Read the model definition and answer for the solid it produces. Units are mm, in the model's axes. A direction names the side the tool comes from. Coordinates: 2 decimals unless noted, no trailing zeros. Loops run counter-clockwise (first coordinate to the right, second up) from the corner with the lowest first, then second, coordinate; pieces in that order, holes last. Notation, with made-up numbers: (30, -10) -> (42, -10) arc R26 ccw to (42, 14) -> close; hole circle Ø11 at (-6.5, -18.75). An arc over 180 degrees is marked (long way). Answer as a JSON object with one key per item and string values. Group by question number.
1) Consider probe 1 along Z at (x, y) = (66.25, -11); probe 2 along Z at (x, y) = (66.5, -12.5); probe 3 along Y at (x, z) = (70.75, 12.5). Determine where each line is inside the solid, lowest interval first. Write a range as [from, to].
2) Section A-A, the plane z = -61.5 is taken. Give the vertices of the cut face in (x, y), plus the area to 3 significant figures.
3) Section C-C, the plane z = -37.5 is taken. Give the vertices of the cut face in (x, y), plus the area to 3 significant figures.
4) Which of the six approach directions +Z, -Z, +X, -X, +Y, -Y give full straight-line access (tool end or side, diameter ignored) to faces 1 (the face through (67.438, -19.529, -39.122)), 2 (the face through (71, -18, -17.546)), 3 (the face through (69.563, -27.304, -67.9))?
5) Flat-ended cylindrical pins translate along their axes: P1, Ø2, axis at x = 69.5, y = -17.5, coming from the +Z side; P2, Ø1.5, axis at x = 67, z = -55, coming from the -Y side; P3, Ø1.5, axis at x = 69, z = -9.5, coming from the -Y side. Find the tip coordinate at first contact, or state that the pin passes through.
6) Determine the mould class of faces 4 (the face through (69, 0, 5)), 5 (the face through (71, -19.393, -2)) for opening direction Z: released by +Z, released by -Z, zero draft, split by the parting line, or undercut.
7) Section B-B, the plane y = -21 is taken. Give the vertices of the cut face in (x, z), plus the area to 3 significant figures.
from build123d import *

# Parameters (mm, degrees)
F1_DEPTH    = 37
F2_T1_DEPTH = 342.8505669038
F3_T        = -2.54
F4_W        = 125.55387271
F4_H        = 111.9176980871
F5_DEPTH    = 25.4
F6_R        = 3.175
F7_DEPTH    = 19.05
F9_DEPTH    = 142.24
F10_W       = 3.5
F10_H       = 32
F11_DEPTH   = 5
F12_W       = 142.5411626697
F12_H       = 154.7065079212
F13_DEPTH   = 37.001


# Not quite as in the source:
# - a fillet or chamfer that OpenCascade refuses, or shapes differently, is made with other operations: its cross-section is extruded or revolved along the edge and cut away or added


with BuildPart() as f1:
    # F0 (on Front) → F1 (new body)
    with BuildSketch(Plane.XZ):
        with BuildLine():
            Line((62.5, 75.5), (-72.5, 75.5))
            Line((-72.5, 75.5), (-72.5, -75.5))
            Line((-72.5, -75.5), (62.5, -75.5))
            ThreePointArc((62.5, -75.5), (69.5710678119, -72.5710678119), (72.5, -65.5))
            Line((72.5, -65.5), (72.5, 65.5))
            ThreePointArc((72.5, 65.5), (69.5710678119, 72.5710678119), (62.5, 75.5))
        make_face()
    extrude(amount=F1_DEPTH)

    # F2: chamfer of 40 x 8 on 1 edges, made by hand

    # F2_s2 → F2_t1 (cut)
    with BuildSketch(Plane.YZ.offset(-176.4252834519)):
        Polygon((-40, -75.5), (0, -67.5), (0, -75.5), align=None)
    extrude(amount=F2_T1_DEPTH, mode=Mode.SUBTRACT)

    # F3
    f3_openings = [f1.faces().sort_by_distance(p)[0] for p in [
        (-0.123954, -37, 0.284541),
    ]]
    offset(amount=F3_T, openings=f3_openings)

    # F4 (on face) → F5 (cut)
    with BuildSketch(Plane.XZ.offset(2.54)):
        with Locations((-0.276936355, 9.5411509565)):
            Rectangle(F4_W, F4_H)
    extrude(amount=-F5_DEPTH, mode=Mode.SUBTRACT)

    # F6 (on face) → F7 (cut)
    with BuildSketch(Plane(origin=(-72.5, 0, 0), x_dir=(0, -1, 0), z_dir=(-1, 0, 0))):
        with Locations((21.3561020792, 0)):
            Circle(F6_R)
        with Locations((21.3561020792, 35)):
            Circle(F6_R)
        with Locations((21.3561020792, -30)):
            Circle(F6_R)
    extrude(amount=-F7_DEPTH, mode=Mode.SUBTRACT)

    # F8 (on face) → F9 (join)
    with BuildSketch(Plane(origin=(69.96, 0, 0), x_dir=(0, -1, 0), z_dir=(-1, 0, 0))):
        Polygon((0, -28.8742875891), (37, -48.2893098931), (37, -45.4208615419), (0, -26.005839238), align=None)
        Polygon((0, -2.637839238), (37, -22.0528615419), (37, -19.1844131908), (0, 0.2306091132), align=None)
        Polygon((0, 23.5986091132), (37, 4.1835868092), (37, 7.0520351604), (0, 26.4670574643), align=None)
        Polygon((0, 49.8350574643), (37, 30.4200351604), (37, 33.2884835115), (0, 52.7035058155), align=None)
    extrude(amount=F9_DEPTH)

    # F10 (on face) → F11 (cut)
    with BuildSketch(Plane.YZ.offset(72.5)):
        with Locations((-17.6429149747, -1.5458973408)):
            Rectangle(F10_W, F10_H)
    extrude(amount=-F11_DEPTH, mode=Mode.SUBTRACT)

    # F12 (on face) → F13 (cut, through all)
    with BuildSketch(Plane.XZ.offset(37)):
        with Locations((-6.4269788563, 0.7590651512)):
            Rectangle(F12_W, F12_H)
    extrude(amount=-F13_DEPTH, mode=Mode.SUBTRACT)


solid = f1.part
Determined:
{
 "1": {"probe 1": "[-69.7, -67.11], [-34.65, -31.78], [-8.41, -5.54], [17.83, 20.7], [44.06, 46.93], [71.95, 74.77]", "probe 2": "[-70, -67.41], [-35.43, -32.56], [-9.2, -6.33], [17.04, 19.91], [43.28, 46.14], [71.8, 74.67]", "probe 3": "[-37, -19.39], [-15.89, 0]"},
 "2": {"outline": "(64.84, -2.54) -> (69.96, -2.54) -> (69.96, -37) -> (72.5, -37) -> (72.5, 0) -> (64.84, 0) -> close", "area": "107 mm²"},
 "3": {"outline": "(64.84, -21.9) -> (69.96, -21.9) -> (69.96, -37) -> (72.5, -37) -> (72.5, 0) -> (64.84, 0) -> (64.84, -2.54) -> (69.96, -2.54) -> (69.96, -16.44) -> (64.84, -16.44) -> close", "area": "135 mm²"},
 "4": {"face 1": "-X", "face 2": "+X, -X", "face 3": "-X, -Y"},
 "5": {"P1": "z = 73.5", "P2": "y = -2.54", "P3": "y = -19.97"},
 "6": {"face 4": "zero draft", "face 5": "undercut"},
 "7": {"outline": "(64.84, -71.7) -> (70.35, -71.7) arc R10 ccw to (72.5, -65.5) -> (72.5, 65.5) arc R10 ccw to (64.84, 75.22) -> (64.84, 72.58) arc R7.46 cw to (69.96, 65.5) -> (69.96, 41.68) -> (64.84, 41.68) -> (64.84, 38.82) -> (69.96, 38.82) -> (69.96, 15.45) -> (64.84, 15.45) -> (64.84, 12.58) -> (69.96, 12.58) -> (69.96, -10.79) -> (64.84, -10.79) -> (64.84, -13.66) -> (69.96, -13.66) -> (69.96, -37.03) -> (64.84, -37.03) -> (64.84, -39.89) -> (69.96, -39.89) -> (69.96, -65.5) arc R7.46 cw to (69.03, -69.11) -> (64.84, -69.11) -> close", "area": "446 mm²"}
}
